```python
from build123d import *

# Parameters (mm, degrees)
SKETCH_1_R          = 22
SKETCH_1_R_2        = 2
EXTRUDE_1_DEPTH     = 3
SKETCH_2_R          = 3
CUT_EXTRUDE_1_DEPTH = 3
SKETCH_4_R          = 1.550336064
SKETCH_4_R_2        = 1.6
CUT_EXTRUDE_2_DEPTH = 3
SKETCH_5_R          = 1.6
CUT_EXTRUDE_3_DEPTH = 3
SKETCH_6_R          = 1.6
CUT_EXTRUDE_4_DEPTH = 3
SKETCH_7_R          = 1.6
CUT_EXTRUDE_7_DEPTH = 149.01191544


with BuildPart() as part:
    # 草图1 → 凸台-拉伸1 (new body)
    with BuildSketch(Plane(origin=(0, 0, -47.111716595), x_dir=(-1, 0, 0), z_dir=(0, 0, -1))):
        Polygon((-65.204960674, 2.259155248), (25.815510263, 2.259155248), (80.848097232, 42.139739941), (80.848097232, 93.718256609), (56.600680459, 115.359857107), (-11.322058774, 115.359857107), (-92.685654124, 56.364707651), (-92.685654124, 19.698826092), align=None)
        with Locations((-2.976767055, 49.573611164)):
            Circle(SKETCH_1_R, mode=Mode.SUBTRACT)
        with Locations((22.138317691, 35.074213997)):
            Circle(SKETCH_1_R_2, mode=Mode.SUBTRACT)
    extrude(amount=EXTRUDE_1_DEPTH)

    # 草图2 → 切除-拉伸1 (cut)
    with BuildSketch(Plane(origin=(0, 0, -50.111716595), x_dir=(-1, 0, 0), z_dir=(0, 0, -1))):
        with Locations((47.733232945, 99.733611164)):
            Circle(SKETCH_2_R)
    extrude(amount=-CUT_EXTRUDE_1_DEPTH, mode=Mode.SUBTRACT)

    # 草图4 → 切除-拉伸2 (cut)
    with BuildSketch(Plane(origin=(0, 0, -50.111716595), x_dir=(-1, 0, 0), z_dir=(0, 0, -1))):
        with Locations((21.127768308, 20.846944547)):
            Circle(SKETCH_4_R)
        with Locations((-2.976767055, 12.073611164)):
            Circle(SKETCH_4_R)
        with Locations((-27.081302418, 20.846944547)):
            Circle(SKETCH_4_R)
        with Locations((-39.907057793, 43.061804502)):
            Circle(SKETCH_4_R)
        with Locations((-35.452719697, 68.323611164)):
            Circle(SKETCH_4_R)
        with Locations((-15.802522429, 84.812084444)):
            Circle(SKETCH_4_R)
        with Locations((9.84898832, 84.812084444)):
            Circle(SKETCH_4_R)
        with Locations((29.499185587, 68.323611164)):
            Circle(SKETCH_4_R)
        with Locations((33.953694149, 43.062771337)):
            Circle(SKETCH_4_R)
        with Locations((-57.204960674, 9.259155248)):
            Circle(SKETCH_4_R_2)
        with Locations((-39.204960674, 9.259155248)):
            Circle(SKETCH_4_R_2)
    extrude(amount=-CUT_EXTRUDE_2_DEPTH, mode=Mode.SUBTRACT)

    # 草图5 → 切除-拉伸3 (cut)
    with BuildSketch(Plane(origin=(0, 0, -50.111716595), x_dir=(-1, 0, 0), z_dir=(0, 0, -1))):
        with Locations((73.848097232, 72.218256609)):
            Circle(SKETCH_5_R)
        with Locations((73.848097232, 64.218256609)):
            Circle(SKETCH_5_R)
    extrude(amount=-CUT_EXTRUDE_3_DEPTH, mode=Mode.SUBTRACT)

    # 草图6 → 切除-拉伸4 (cut)
    with BuildSketch(Plane(origin=(0, 0, -50.111716595), x_dir=(-1, 0, 0), z_dir=(0, 0, -1))):
        with Locations((-82.099946385, 55.393733062)):
            Circle(SKETCH_6_R)
        with Locations((-67.527515299, 65.959917436)):
            Circle(SKETCH_6_R)
        with Locations((-28.262054197, 94.430534254)):
            Circle(SKETCH_6_R)
        with Locations((-13.689623111, 104.996718629)):
            Circle(SKETCH_6_R)
    extrude(amount=-CUT_EXTRUDE_4_DEPTH, mode=Mode.SUBTRACT)

    # 草图7 → 切除-拉伸7 (cut, through all)
    with BuildSketch(Plane(origin=(0, 0, -50.111716595), x_dir=(-1, 0, 0), z_dir=(0, 0, -1))):
        with Locations((12.815510263, 9.259155248)):
            Circle(SKETCH_7_R)
        with Locations((20.815510263, 9.259155248)):
            Circle(SKETCH_7_R)
    extrude(amount=-CUT_EXTRUDE_7_DEPTH, mode=Mode.SUBTRACT)


solid = part.part
```
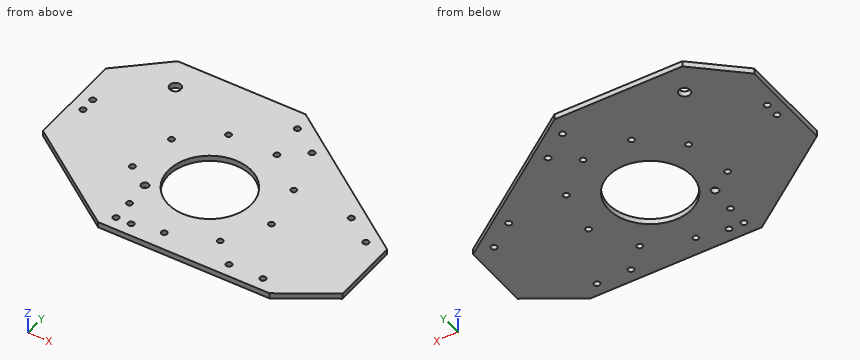
Could you check a few things on this model? Use its own coordinates, in mm. Give positions to 0.01 mm unless a question says otherwise; leave off trailing zeros. Order: outer loops, then holes, each group sorted by start corner. A loop starts at its lowest first (then second) coordinate and runs counter-clockwise, first axis right, second up.
Q1. Suppose I cut it at D-D, the plane x = -39. Write out the boundary of the cut face in (y, z), and give its area (3 significant figures).
Q2. Suppose I cut it at B-B, the plane z = -47.9. Count the separate pieces of the cut face and the enclosed holes in it, and give its area (3 significant figures).
Q3. Suppose I cut it at C-C, the plane y = 59. Write out the boundary of the cut face in (x, z).
Q4. Suppose I cut it at A-A, the plane y = 29.5. Write out the boundary of the cut face in (x, z).
Q5. I'm going to push flat-ended pins straight in: P1, Ø1.5, axis at y = 74.5, z = -49.5, coming from the +X side; P2, Ø3.5, axis at x = -22.14, y = 35.07, coming from the -Z side; P3, Ø1, axis at y = 22, z = -49, coming from the -X side; P4, Ø1.5, axis at x = 74.5, z = -49, coming from the -Y side. Where does each tip first touch, or does it pass through?
Q6. If I drill on line 1 along Y through (x, z) = (-12.5, -47.5); line 2 along X through (y, z) = (85.5, -49.4); line 3 along Y through (x, z) = (4, -47.4), over which ranges is the centre line in solid material (lowest first)?
Solution:
1. outline: (11.81, -50.11) - (115.36, -50.11) - (115.36, -47.11) - (11.81, -47.11) - close
1. area: 311 mm2
2. separate pieces: 1
2. enclosed holes: 22
2. area: 13,900 mm2
3. outline: (-80.85, -50.11) - (-16.9, -50.11) - (-16.9, -47.11) - (-80.85, -47.11) - close; (22.85, -50.11) - (89.05, -50.11) - (89.05, -47.11) - (22.85, -47.11) - close
4. outline: (-63.41, -50.11) - (-6.03, -50.11) - (-6.03, -47.11) - (-63.41, -47.11) - close; (11.98, -50.11) - (92.69, -50.11) - (92.69, -47.11) - (11.98, -47.11) - close
5. P1: stops at x = 68.71
5. P2: passes through
5. P3: stops at x = -53.75
5. P4: stops at y = 7.68
6. line 1: y = 2.26 to 7.69, 10.83 to 33.94, 65.21 to 115.36
6. line 2: x = -80.85 to -11.24, -8.46 to 14.41, 17.19 to 52.5
6. line 3: y = 2.26 to 10.91, 13.24 to 27.6, 71.55 to 115.36
